Check sheet for the modelled part. Datum: model origin and axes. Units: mm. A direction names the side the tool comes from. Coordinates: 2 decimals unless noted, no trailing zeros. Write each loop counter-clockwise with the first axis right and the second up, starting at its lowest first coordinate (ties: lowest second). Pieces come first, ordered by that corner, then holes. Notation, with made-up numbers: (-23.75, -37.5) - (-15.75, -37.5) arc R22 cw to (-15.75, -25.5) - close; hole circle Ø5 at (-15, 78.25). An arc over 180 degrees is marked (long way). Use one line per item in the form item = value. Start each with the question number.
1. Go/stop test with flat-tipped pins: pin 1 Ø1 at (y, z) = (9, 14.5) entering from +X; pin 2 Ø3 at (x, y) = (43, 1.5) entering from -Z; pin 3 Ø1 at (x, y) = (19, 3) entering from +Z; pin 4 Ø0.6 at (x, z) = (2, 19.5) entering from +Y. Record where each tip stops, or that it passes through.
2. Cross-section at B-B on y = 7.75. Record the boundary of the cut face in (x, z).
3. Cross-section at C-C on z = 22.5. Give the number of separate pieces and of enclosed holes in the cut face, then the cut area to 3 significant figures.
4. Cross-section at D-D on x = 48.5. Record the boundary of the cut face in (y, z), then the cut area to 3 significant figures.
5. Tool access check on faces 1 (the face through (27, 0, 12)), 2 (the face through (52, 1.3, 22)). Record the directions out of +Z, -Z, +X, -X, +Y, -Y that give a thin tool (end or side, any length) a straight path to the whole face; none if there is none.
6. Draft check along Z on faces 3 (the face through (1, 1.3, 22)), 4 (the face through (0, 1, 12)), 5 (the face through (27, 1, 0)). Enter one of: +Z half, -Z half, draft (parallel to the pull), parting line (faces both ways), or undercut.
7. Scan lines: line 1 along Z through (x, y) = (52.5, 0.95); line 2 along Z through (x, y) = (44.3, 0.6); line 3 along Z through (x, y) = (9, 1.15). Record each from-to range of solid material in increasing order.
```python
from build123d import *

# Parameters (mm, degrees)
SKETCH1_W           = 54
SKETCH1_H           = 24
BOSS_EXTRUDE1_DEPTH = 1.5
CUT_EXTRUDE1_REACH  = 3.5
SKETCH2_R           = 1.5
SKETCH4_W           = 3
SKETCH4_H           = 3
CUT_EXTRUDE2_DEPTH  = 0.2
CUT_EXTRUDE3_REACH  = 3.5
SKETCH5_R           = 0.5
CUT_EXTRUDE4_DEPTH  = 0.1
CUT_EXTRUDE5_DEPTH  = 0.1
SKETCH10_R          = 5
BOSS_EXTRUDE2_DEPTH = 10
FILLET1_R           = 1


with BuildPart() as part:
    # Sketch1 → Boss-Extrude1 (new body)
    with BuildSketch(Plane(origin=(0, 0, 0), x_dir=(1, 0, 0), z_dir=(0, 1, 0))):
        with Locations((27, -12)):
            Rectangle(SKETCH1_W, SKETCH1_H)
    extrude(amount=BOSS_EXTRUDE1_DEPTH)

    # Sketch2 → Cut-Extrude1 (cut, up to next)
    with BuildSketch(Plane(origin=(0, 1.5, 0), x_dir=(1, 0, 0), z_dir=(0, 1, 0)), mode=Mode.PRIVATE) as cut_extrude1_sk1:
        with Locations((9, -2.5)):
            Circle(SKETCH2_R)
    cut_extrude1_tool1 = extrude(cut_extrude1_sk1.sketch, amount=-CUT_EXTRUDE1_REACH, mode=Mode.PRIVATE) & part.part
    add(cut_extrude1_tool1.solids().sort_by_distance((9, 1.5, 2.5))[0], mode=Mode.SUBTRACT)
    # Sketch2 → Cut-Extrude1 (cut, up to next)
    with BuildSketch(Plane(origin=(0, 1.5, 0), x_dir=(1, 0, 0), z_dir=(0, 1, 0)), mode=Mode.PRIVATE) as cut_extrude1_sk2:
        with Locations((44.3, -21.5)):
            Circle(SKETCH2_R)
    cut_extrude1_tool2 = extrude(cut_extrude1_sk2.sketch, amount=-CUT_EXTRUDE1_REACH, mode=Mode.PRIVATE) & part.part
    add(cut_extrude1_tool2.solids().sort_by_distance((44.3, 1.5, 21.5))[0], mode=Mode.SUBTRACT)

    # Sketch4 → Cut-Extrude2 (cut)
    with BuildSketch(Plane(origin=(0, 1.5, 0), x_dir=(1, 0, 0), z_dir=(0, 1, 0))):
        with Locations((1.51, -1.51)):
            Rectangle(SKETCH4_W, SKETCH4_H)
        with Locations((52.49, -1.51)):
            Rectangle(SKETCH4_W, SKETCH4_H)
        with Locations((1.51, -22.49)):
            Rectangle(SKETCH4_W, SKETCH4_H)
        with Locations((52.49, -22.49)):
            Rectangle(SKETCH4_W, SKETCH4_H)
    extrude(amount=-CUT_EXTRUDE2_DEPTH, mode=Mode.SUBTRACT)

    # Sketch5 → Cut-Extrude3 (cut, up to next)
    with BuildSketch(Plane.XZ, mode=Mode.PRIVATE) as cut_extrude3_sk1:
        with Locations((52.5, 1.5)):
            Circle(SKETCH5_R)
    cut_extrude3_tool1 = extrude(cut_extrude3_sk1.sketch, amount=-CUT_EXTRUDE3_REACH, mode=Mode.PRIVATE) & part.part
    add(cut_extrude3_tool1.solids().sort_by_distance((52.5, 0, 1.5))[0], mode=Mode.SUBTRACT)
    # Sketch5 → Cut-Extrude3 (cut, up to next)
    with BuildSketch(Plane.XZ, mode=Mode.PRIVATE) as cut_extrude3_sk2:
        with Locations((52.5, 22.5)):
            Circle(SKETCH5_R)
    cut_extrude3_tool2 = extrude(cut_extrude3_sk2.sketch, amount=-CUT_EXTRUDE3_REACH, mode=Mode.PRIVATE) & part.part
    add(cut_extrude3_tool2.solids().sort_by_distance((52.5, 0, 22.5))[0], mode=Mode.SUBTRACT)
    # Sketch5 → Cut-Extrude3 (cut, up to next)
    with BuildSketch(Plane.XZ, mode=Mode.PRIVATE) as cut_extrude3_sk3:
        with Locations((1.5, 1.5)):
            Circle(SKETCH5_R)
    cut_extrude3_tool3 = extrude(cut_extrude3_sk3.sketch, amount=-CUT_EXTRUDE3_REACH, mode=Mode.PRIVATE) & part.part
    add(cut_extrude3_tool3.solids().sort_by_distance((1.5, 0, 1.5))[0], mode=Mode.SUBTRACT)
    # Sketch5 → Cut-Extrude3 (cut, up to next)
    with BuildSketch(Plane.XZ, mode=Mode.PRIVATE) as cut_extrude3_sk4:
        with Locations((1.5, 22.5)):
            Circle(SKETCH5_R)
    cut_extrude3_tool4 = extrude(cut_extrude3_sk4.sketch, amount=-CUT_EXTRUDE3_REACH, mode=Mode.PRIVATE) & part.part
    add(cut_extrude3_tool4.solids().sort_by_distance((1.5, 0, 22.5))[0], mode=Mode.SUBTRACT)

    # Sketch8 → Cut-Extrude4 (cut)
    with BuildSketch(Plane(origin=(0, 1.5, 0), x_dir=(1, 0, 0), z_dir=(0, 1, 0))):
        Polygon((0.556961838, -3.555375385), (0.73765094, -3.555375385), (0.457202222, -5.555375385), (0.27651312, -5.555375385), align=None)
        Polygon((2.58140094, -3.555375385), (2.762090043, -3.555375385), (2.481641325, -5.555375385), (2.438372094, -5.555375385), (1.321384915, -3.96362859), (1.098227863, -5.555375385), (0.917538761, -5.555375385), (1.197987479, -3.555375385), (1.24125671, -3.555375385), (2.357843248, -5.146721539), align=None)
        Polygon((3.635487479, -4.478452308), (3.635487479, -3.888708718), (3.814974658, -3.888708718), (3.814974658, -4.478452308), (4.404718248, -4.478452308), (4.404718248, -4.657939488), (3.814974658, -4.657939488), (3.814974658, -5.247683077), (3.635487479, -5.247683077), (3.635487479, -4.657939488), (3.045743889, -4.657939488), (3.045743889, -4.478452308), align=None)
    extrude(amount=-CUT_EXTRUDE4_DEPTH, mode=Mode.SUBTRACT)

    # Sketch9 → Cut-Extrude5 (cut)
    with BuildSketch(Plane(origin=(0, 1.5, 0), x_dir=(1, 0, 0), z_dir=(0, 1, 0))):
        Polygon((0.519157464, -18.562132586), (0.699846567, -18.562132586), (0.419397849, -20.562132586), (0.238708746, -20.562132586), align=None)
        Polygon((2.543596567, -18.562132586), (2.724285669, -18.562132586), (2.443836951, -20.562132586), (2.40056772, -20.562132586), (1.283580541, -18.970385792), (1.06042349, -20.562132586), (0.879734387, -20.562132586), (1.160183105, -18.562132586), (1.203452336, -18.562132586), (2.320038874, -20.15347874), align=None)
        Polygon((2.8769299, -19.741619766), (3.623324131, -19.741619766), (3.598885028, -19.921106945), (2.854093361, -19.921106945), align=None)
    extrude(amount=-CUT_EXTRUDE5_DEPTH, mode=Mode.SUBTRACT)

    # Sketch10 → Boss-Extrude2 (add)
    with BuildSketch(Plane(origin=(0, 1.5, 0), x_dir=(1, 0, 0), z_dir=(0, 1, 0))):
        with Locations((5.5, -12)):
            Circle(SKETCH10_R)
        with Locations((48.5, -12)):
            Circle(SKETCH10_R)
    extrude(amount=BOSS_EXTRUDE2_DEPTH)

    # Fillet1
    fillet1_edges = [part.edges().sort_by_distance(p)[0] for p in [
        (0.5, 11.5, 12),
        (43.5, 11.5, 12),
    ]]
    fillet(fillet1_edges, radius=FILLET1_R)


solid = part.part
```
Final values:
q1.pin_1 = 53.08
q1.pin_2 = 0
q1.pin_3 = through
q1.pin_4 = 1.5
q2.outline = circle Ø10 at (5.5, 12); circle Ø10 at (48.5, 12)
q3.separate_pieces = 4
q3.enclosed_holes = 0
q3.area = 73.8 mm²
q4.outline = (0, 0) - (1.5, 0) - (1.5, 7) - (10.5, 7) arc R1 ccw to (11.5, 8) - (11.5, 16) arc R1 ccw to (10.5, 17) - (1.5, 17) - (1.5, 24) - (0, 24) - close
q4.area = 136 mm²
q5.face_1 = +Z, -Z, +X, -X, -Y
q5.face_2 = +Y
q6.face_3 = undercut
q6.face_4 = draft
q6.face_5 = -Z half
q7.line_1 = 0 to 1, 2 to 22, 23 to 24
q7.line_2 = 0 to 20, 23 to 24
q7.line_3 = 0 to 1, 4 to 24
